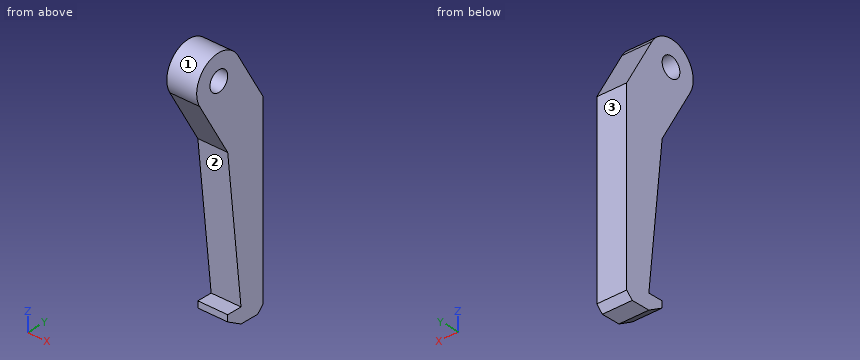
Autodesk Inventor part; units mm, degrees
ref_plane "YZ Plane" through (0, 0, 0) normal (1, 0, 0) x (0, 1, 0)
ref_plane "XZ Plane" through (0, 0, 0) normal (0, 1, 0) x (-1, 0, 0)
ref_plane "XY Plane" through (0, 0, 0) normal (0, 0, 1) x (1, 0, 0)
sketch "Skizze1" plane through (0, 0, 0) normal (1, 0, 0) x (0, 1, 0)
  line L0 (-88.8183, 0) -> (21.3265, 0)
  line L1 (0, -72.4192) -> (0, 123.5808)
  line L2 (-61.844, -44.4192) -> (-61.844, 95.5808)
  line L3 (-31.844, 50.9398) -> (-31.844, -24.4192)
  line L4 (-41.844, -18.4192) -> (-47.844, -18.4192)
  line L5 (-41.844, -24.4192) -> (-47.844, -20.9551)
  line L6 (-41.844, -24.4192) -> (-34.9129, -24.4192) construction
  line L7 (-31.844, 50.9398) -> (-43.1838, 70.5808)
  line L8 (-31.844, 50.9398) -> (-5.6477, 50.9398) construction
  circle A0 centre (-51.844, 65.5808) radius 10
  line L9 (-60.5043, 60.5808) -> (-47.844, 38.6526)
  line L10 (-61.844, 62.7769) -> (-45.1591, 62.7769) construction
  line L11 (-47.844, 38.6526) -> (-41.844, -18.4192)
  line L12 (-31.844, -24.4192) -> (-41.844, -24.4192)
  line L13 (-47.844, -20.9551) -> (-47.844, -18.4192)
  line L14 (-73.0833, 75.5808) -> (5.5916, 75.5808)
  point P0 (0, 0)
  point P1 (-61.844, 75.5808)
  point P2 (-37.5139, 60.7603)
  dimension "d0" = 150
  dimension "d1" = 120
  dimension "d2" = 60
  dimension "d3" = 6
  dimension "d4" = 16
  dimension "d5" = 10
  dimension "d6" = 20
  dimension "d7" = 30
  dimension "d8" = 16
extrude "Extrusion1" add sketch "Skizze1" along normal blind 12 contours L11 L9 A0 L7 L3 L0 | L0 L3 L12 L5 L13 L4 L11 | A0
hole "Bohrung1" at (0, -51.844, 65.5808) direction (1, 0, 0) diameter 8 end through all
chamfer "Fasen1" distance 2.5 angle 45 1 edges at (6, -31.844, -24.4192) measured on face at (4, -38.5107, -24.4192)
properties part number "Abzieher_Klaue1" material "1.0038 S235JR"
Design review of the part built by this model. Coordinates are the model's own, in mm. Face numbers are marked on the shaded views. Give positions to 0.01 mm unless a question says otherwise; leave off trailing zeros. Loops run counter-clockwise (first coordinate to the right, second up) from the corner with the lowest first, then second, coordinate; pieces in that order, holes last. Notation, with made-up numbers: (-24.75, 56.25) -> (27.25, 56.25) arc R17 cw to (27.25, 80.25) -> close; hole circle Ø6 at (63, -7.75). An arc over 180 degrees is marked (long way). One line per item, written item: value.
Q1. Draft analysis for pull direction Z (two halves, no side actions). For the marked faces 1, 2 and 3, state which applies: pulls with the +Z half, pulls with the -Z half, needs draft (parallel to the pull), parting line crosses it, or undercut.
Numbers:
face 1: parting line crosses it
face 2: undercut
face 3: needs draft
Q2. For pin 1 Ø1 at (x, z) = (4.5, 26) entering from -Y; pin 2 Ø6.5 at (x, y) = (3, -44) entering from +Z; pin 3 Ø1.5 at (y, z) = (-36, 60) entering from -X (3 decimals); pin 4 Ø1.5 at (x, z) = (5, 57.5) entering from -Y, all flat-tipped, find the tip position at first contact; note any pin that passes through.
Numbers:
pin 1: stops at y = -46.57
pin 2: stops at z = 74.46
pin 3: passes through
pin 4: stops at y = -59.16
Q3. We need section D-D on z = -13.5. Give the boundary of the cut face in (x, y).
Numbers:
outline: (0, -42.36) -> (12, -42.36) -> (12, -31.84) -> (0, -31.84) -> close
Q4. For L1, parallel to Z at x = 1.5, y = -49; L2, parallel to Z at x = 5, y = -55; L3, parallel to Y at x = 1.5, z = 6, list the stretches that pass through material, from the lowest coordinate up.
Numbers:
L1: z = 40.65 to 62.77, 68.39 to 75.17
L2: z = 51.05 to 63.12, 68.04 to 75.07
L3: y = -44.41 to -31.84
Q5. We need section B-B on z = 68. Give the boundary of the cut face in (x, y).
Numbers:
outline: (0, -61.55) -> (12, -61.55) -> (12, -55.03) -> (0, -55.03) -> close; (0, -48.66) -> (12, -48.66) -> (12, -41.69) -> (0, -41.69) -> close
Q6. We need section C-C on x = 7.5. Give the boundary of the cut face in (y, z).
Numbers:
outline: (-60.5, 60.58) -> (-47.84, 38.65) -> (-41.84, -18.42) -> (-47.84, -18.42) -> (-47.84, -20.96) -> (-41.84, -24.42) -> (-34.34, -24.42) -> (-31.84, -21.92) -> (-31.84, 50.94) -> (-43.18, 70.58) arc R10 ccw to start; hole circle Ø8 at (-51.84, 65.58)
Q7. We need section A-A on y = -52.75. Give the boundary of the cut face in (x, z), and give its area (3 significant figures).
Numbers:
outline: (0, 47.15) -> (12, 47.15) -> (12, 61.68) -> (0, 61.68) -> close; (0, 69.48) -> (12, 69.48) -> (12, 75.54) -> (0, 75.54) -> close
area: 247 mm^2
